```python
from build123d import *

# Parameters (mm, degrees)
ESQUISSE1_W             = 10.75
ESQUISSE1_H             = 10.75
BOSS_EXTRU_1_DEPTH      = 10
BOSS_EXTRU_1_2_DEPTH    = 10
ESQUISSE3_W             = 90
ESQUISSE3_H             = 10
BOSS_EXTRU_2_DEPTH      = 5
ESQUISSE4_R             = 2.75
ENL_V_MAT_EXTRU_1_DEPTH = 1.5
CONG_1_R                = 0.5


with BuildPart() as part:
    # Esquisse1 → Boss.-Extru.1 (new body)
    with BuildSketch(Plane.XY):
        with Locations((-39.625, 5.375)):
            Rectangle(ESQUISSE1_W, ESQUISSE1_H)
    extrude(amount=BOSS_EXTRU_1_DEPTH)



with BuildPart() as body_2:
    # Esquisse1 → Boss.-Extru.1 2 (new body)
    with BuildSketch(Plane.XY):
        with Locations((39.625, 5.375)):
            Rectangle(ESQUISSE1_W, ESQUISSE1_H)
    extrude(amount=BOSS_EXTRU_1_2_DEPTH)


with BuildPart() as part_1:
    add(part.part)

    add(body_2.part)  # Boss.-Extru.2 merges body 2
    # Esquisse3 → Boss.-Extru.2 (add)
    with BuildSketch(Plane.XZ):
        with Locations((0, 5)):
            Rectangle(ESQUISSE3_W, ESQUISSE3_H)
    extrude(amount=BOSS_EXTRU_2_DEPTH)

    # Esquisse4 → Enlèv. mat.-Extru.1 (cut)
    with BuildSketch(Plane(origin=(-34.25, 0, 0), x_dir=(0, 0, -1), z_dir=(1, 0, 0))):
        with Locations((-7, 7)):
            Circle(ESQUISSE4_R)
    enl_v_mat_extru_1 = extrude(amount=-ENL_V_MAT_EXTRU_1_DEPTH, mode=Mode.SUBTRACT)

    # Symétrie1: Enlèv. mat.-Extru.1 across plane
    add(enl_v_mat_extru_1.mirror(Plane(origin=(0, 0, 0), x_dir=(0, 0, 1), z_dir=(1, 0, 0))), mode=Mode.SUBTRACT)

    # Congé1
    # the kernel refuses this fillet: 0.5 mm, written as the material it adds along each edge
    with BuildSketch(Plane(origin=(34.25, 0, 0), x_dir=(-1, 0, 0), z_dir=(0, 0, 1)), Plane(origin=(-34.25, 0, 0), x_dir=(0, 1, 0), z_dir=(0, 0, 1))) as cong_1_piece_1:
        with BuildLine():
            CenterArc((CONG_1_R, -CONG_1_R), CONG_1_R, 90, 90)
            Line((0, -CONG_1_R), (0, 0))
            Line((0, 0), (CONG_1_R, 0))
        make_face()
    extrude(amount=10)
    # the kernel refuses this fillet: 0.5 mm, written as the material it takes off along each edge
    with BuildSketch(Plane(origin=(33.75, 0, 0), x_dir=(0, -1, 0), z_dir=(-1, 0, 0)), Plane(origin=(-33.75, 0, 10), x_dir=(0, -1, 0), z_dir=(1, 0, 0))) as cong_1_2_piece_1:
        with BuildLine():
            CenterArc((CONG_1_R, CONG_1_R), CONG_1_R, 180, 90)
            Line((0, CONG_1_R), (0, 0))
            Line((0, 0), (CONG_1_R, 0))
        make_face()
    extrude(amount=67.5, mode=Mode.SUBTRACT)
    with BuildSketch(Plane(origin=(34.25, 12, 0), x_dir=(1, 0, 0), z_dir=(0, -1, 0)), Plane(origin=(-34.25, 0.5, 10), x_dir=(0, 0, -1), z_dir=(0, 1, 0))) as cong_1_2_piece_2:
        with BuildLine():
            CenterArc((CONG_1_R, CONG_1_R), CONG_1_R, 180, 90)
            Line((0, CONG_1_R), (0, 0))
            Line((0, 0), (CONG_1_R, 0))
        make_face()
    extrude(amount=11.5, mode=Mode.SUBTRACT)
    with BuildSketch(Plane(origin=(34.25, 10.75, -1.25), x_dir=(1, 0, 0), z_dir=(0, 0, 1)), Plane(origin=(45, 10.75, -1.25), x_dir=(0, -1, 0), z_dir=(0, 0, 1)), Plane(origin=(-45, 10.75, -1.25), x_dir=(1, 0, 0), z_dir=(0, 0, 1))) as cong_1_2_piece_3:
        with BuildLine():
            CenterArc((CONG_1_R, -CONG_1_R), CONG_1_R, 90, 90)
            Line((0, -CONG_1_R), (0, 0))
            Line((0, 0), (CONG_1_R, 0))
        make_face()
    extrude(amount=12.5, mode=Mode.SUBTRACT)
    with BuildSketch(Plane(origin=(34.25, 12, 10), x_dir=(1, 0, 0), z_dir=(0, -1, 0)), Plane(origin=(-34.25, 0.5, 0), x_dir=(0, 0, 1), z_dir=(0, 1, 0))) as cong_1_2_piece_4:
        with BuildLine():
            CenterArc((CONG_1_R, -CONG_1_R), CONG_1_R, 90, 90)
            Line((0, -CONG_1_R), (0, 0))
            Line((0, 0), (CONG_1_R, 0))
        make_face()
    extrude(amount=11.5, mode=Mode.SUBTRACT)
    with BuildSketch(Plane(origin=(-34.25, 10.75, -1.25), x_dir=(-1, 0, 0), z_dir=(0, 0, 1))) as cong_1_2_piece_5:
        with BuildLine():
            CenterArc((CONG_1_R, CONG_1_R), CONG_1_R, 180, 90)
            Line((0, CONG_1_R), (0, 0))
            Line((0, 0), (CONG_1_R, 0))
        make_face()
    extrude(amount=12.5, mode=Mode.SUBTRACT)
    with BuildSketch(Plane(origin=(-33.75, 0.5, 0), x_dir=(-1, 0, 0), z_dir=(0, 1, 0))) as cong_1_2_piece_6:
        with BuildLine():
            CenterArc((0.5 + CONG_1_R, CONG_1_R), CONG_1_R, 180, 90)
            Line((0.5, CONG_1_R), (0.5, 0))
            Line((0.5, 0), (0.5 + CONG_1_R, 0))
        make_face()
    revolve(axis=Axis((-33.75, 0.5, 0), (0, 0, 1)), revolution_arc=90, mode=Mode.SUBTRACT)
    with BuildSketch(Plane(origin=(-33.75, 0.5, 10), x_dir=(-1, 0, 0), z_dir=(0, 1, 0))) as cong_1_2_piece_7:
        with BuildLine():
            CenterArc((0.5 + CONG_1_R, -CONG_1_R), CONG_1_R, 90, 90)
            Line((0.5, -CONG_1_R), (0.5, 0))
            Line((0.5, 0), (0.5 + CONG_1_R, 0))
        make_face()
    revolve(axis=Axis((-33.75, 0.5, 10), (0, 0, 1)), revolution_arc=90, mode=Mode.SUBTRACT)
    with BuildSketch(Plane(origin=(33.75, 0.5, 10), x_dir=(0, -1, 0), z_dir=(-1, 0, 0))) as cong_1_2_piece_8:
        with BuildLine():
            CenterArc((0.5 + CONG_1_R, -CONG_1_R), CONG_1_R, 90, 90)
            Line((0.5, -CONG_1_R), (0.5, 0))
            Line((0.5, 0), (0.5 + CONG_1_R, 0))
        make_face()
    revolve(axis=Axis((33.75, 0.5, 10), (0, 0, 1)), revolution_arc=90, mode=Mode.SUBTRACT)
    with BuildSketch(Plane(origin=(33.75, 0.5, 0), x_dir=(0, -1, 0), z_dir=(-1, 0, 0))) as cong_1_2_piece_9:
        with BuildLine():
            CenterArc((0.5 + CONG_1_R, CONG_1_R), CONG_1_R, 180, 90)
            Line((0.5, CONG_1_R), (0.5, 0))
            Line((0.5, 0), (0.5 + CONG_1_R, 0))
        make_face()
    revolve(axis=Axis((33.75, 0.5, 0), (0, 0, 1)), revolution_arc=90, mode=Mode.SUBTRACT)


solid = part_1.part
```
Read the model definition and answer for the solid it produces. Units are mm, in the model's axes. A direction names the side the tool comes from. Round coordinates to 2 decimals unless told otherwise and drop trailing zeros. Write each loop counter-clockwise with the first axis right and the second up, starting at its lowest first coordinate (ties: lowest second). Pieces come first, ordered by that corner, then holes. Notation, with made-up numbers: (-13, 13) - (43, 13) arc R18 cw to (43, 30) - close; hole circle Ø1 at (-25.75, -20.75). An arc over 180 degrees is marked (long way). One line per item, written item: value.
Q1. Straight lines are drawn through the part: line 1 (X direction, y = 9.5, z = 4.25); line 2 (X direction, y = 6, z = 8); line 3 (Y direction, x = -35.2, z = 7). For each, find the intervals that lie inside material, in ascending order. Write a range as from..to.
The answers:
line 1: x = -45..-34.25, 34.25..45
line 2: x = -45..-35.75, 35.75..45
line 3: y = -5..4.25, 9.75..10.75
Q2. For a pull along Z with two mould halves and no side action, classify faces 1 (the flat face through (45, 3, 5)), 2 (the flat face through (-35.75, 7, 7)), 3 (the flat face through (-1, -1, 0)) as pulls with the +Z half, pulls with the -Z half, needs draft (parallel to the pull), parting line crosses it, or undercut.
The answers:
face 1: needs draft
face 2: undercut
face 3: pulls with the -Z half
Q3. Each of these flat-tipped pins is pushed along its axis until it touches: P1, Ø5, axis at x = -17.5, z = 3.5, coming from the +Y side; P2, Ø4, axis at x = 32.5, z = 8.5, coming from the +Y side. Where does it stop, or does it pass through?
The answers:
P1: stops at y = 0
P2: stops at y = 10.68
Q4. Which of the six approach directions +Z, -Z, +X, -X, +Y, -Y give full straight-line access (tool end or side, diameter ignored) to faces 4 (the flat face through (34.25, 4, 4)), 5 (the cylindrical face through (34.99, 4.56, 5.73)), 6 (the flat face through (-45, 3, 5))?
The answers:
face 4: +Z, -Z, +Y
face 5: none
face 6: +Z, -Z, -X, +Y, -Y
Q5. Find section C-C (x = -16). Determine the outline of the cut face in (y, z).
The answers:
outline: (-5, 0) - (-0.5, 0) arc R0.5 ccw to (0, 0.5) - (0, 9.5) arc R0.5 ccw to (-0.5, 10) - (-5, 10) - close
Q6. Find section A-A (z = 7). Determine the outline of the cut face in (x, y).
The answers:
outline: (-45, -5) - (45, -5) - (45, 10.25) arc R0.5 ccw to (44.5, 10.75) - (34.75, 10.75) arc R0.5 ccw to (34.25, 10.25) - (34.25, 9.75) - (35.75, 9.75) - (35.75, 4.25) - (34.25, 4.25) - (34.25, 0.5) arc R0.5 cw to (33.75, 0) - (-33.75, 0) arc R0.5 cw to (-34.25, 0.5) - (-34.25, 4.25) - (-35.75, 4.25) - (-35.75, 9.75) - (-34.25, 9.75) - (-34.25, 10.25) arc R0.5 ccw to (-34.75, 10.75) - (-44.5, 10.75) arc R0.5 ccw to (-45, 10.25) - close
Q7. Find section B-B (y = 7). Determine the outline of the cut face in (x, z), and give its area (3 significant figures).
The answers:
outline: (-45, 0) - (-34.75, 0) arc R0.5 ccw to (-34.25, 0.5) - (-34.25, 4.25) - (-35.75, 4.25) - (-35.75, 9.75) - (-34.32, 9.75) arc R0.5 ccw to (-34.75, 10) - (-45, 10) - close; (34.25, 0.5) arc R0.5 ccw to (34.75, 0) - (45, 0) - (45, 10) - (34.75, 10) arc R0.5 ccw to (34.32, 9.75) - (35.75, 9.75) - (35.75, 4.25) - (34.25, 4.25) - close
area: 198 mm2
